Design review of the part built by this model. Coordinates are the model's own, in mm. Face numbers are marked on the shaded views. A direction names the side the tool comes from. Round coordinates to 2 decimals unless told otherwise and drop trailing zeros. Write each loop counter-clockwise with the first axis right and the second up, starting at its lowest first coordinate (ties: lowest second). Pieces come first, ordered by that corner, then holes. Notation, with made-up numbers: (62, 42.25) -> (117, 42.25) arc R14 ccw to (117, 59.25) -> close; hole circle Ø9 at (73, 60.5). An arc over 180 degrees is marked (long way). Write item = value, one per line. Start each with the question number.
Item 1: Mouldability with a two-part tool opening along X and no side actions: class the marked faces 3, 4, 5 and 6 as released by +X, released by -X, zero draft, split by the parting line, or undercut.
Item 2: Add section C-C, the plane z = 6.25. State how many separate pieces and enclosed holes the cut face has, then the cut area to 3 significant figures.
Item 3: To check wall thickness, follow L1, parallel to X at y = 20.4, z = 4.25; L2, parallel to X at y = 1.5, z = 6.75; L3, parallel to X at y = 19.5, z = 4.75. State the ranges of each line that lie inside material, in increasing order.
Item 4: Add section B-B, the plane y = -24.5. State the section outline as (x, z) points, then the cut area to 3 significant figures.
Item 5: Machinability: for the marked faces 1 and 2, which of the approach directions +Z, -Z, +X, -X, +Y, -Y give a long, thin tool a straight path to every point of the face, cutting with its end or side? Answer none if there is none.
Item 6: For pin 1 Ø2.5 at (x, y) = (27.2, -31.28) entering from +Z; pin 2 Ø4 at (x, z) = (-13.5, 4) entering from -Y; pin 3 Ø4.5 at (x, y) = (-28.5, 20.5) entering from +Z; pin 4 Ø1.5 at (x, y) = (0, -7) entering from -Z, all flat-tipped, find the tip position at first contact; note any pin that passes through.
Item 7: Add section A-A, the plane x = -4.5. State the section outline as (y, z) points, then the cut area to 3 significant figures.
from build123d import *

# Parameters (mm, degrees)
SKETCH2_R           = 1.5
BOSS_EXTRUDE1_DEPTH = 10.35
BOSS_EXTRUDE2_START = 10.35
SKETCH2_3_R         = 1.5
BOSS_EXTRUDE2_DEPTH = 3
FILLET1_SIZE        = 4
FILLET2_SIZE        = 4
SKETCH7_R           = 2.825
CUT_EXTRUDE1_DEPTH  = 3.5


with BuildPart() as part:
    # Sketch2 → Boss-Extrude1 (new body)
    with BuildSketch(Plane.XY):
        Polygon((-30.92, -35), (-23.9, -35), (-23.9, 18.9), (23.9, 18.9), (23.9, -35), (30.92, -35), (30.92, 24.12), (-30.92, 24.12), align=None)
        with Locations((-27.2, -31.28)):
            Circle(SKETCH2_R, mode=Mode.SUBTRACT)
        with Locations((27.2, -31.28)):
            Circle(SKETCH2_R, mode=Mode.SUBTRACT)
        with Locations((-27.2, 20.4)):
            Circle(SKETCH2_R, mode=Mode.SUBTRACT)
        with Locations((27.2, 20.4)):
            Circle(SKETCH2_R, mode=Mode.SUBTRACT)
    extrude(amount=BOSS_EXTRUDE1_DEPTH)

    # Sketch2<3> → Boss-Extrude2 (add)
    # profile 1 of 2: a face of its own
    with BuildSketch(Plane.XY.offset(BOSS_EXTRUDE2_START)):
        Polygon((-30.92, -35), (-23.9, -35), (-23.9, 18.9), (23.9, 18.9), (23.9, -35), (30.92, -35), (30.92, 24.12), (-30.92, 24.12), align=None)
        with Locations((-27.2, -31.28)):
            Circle(SKETCH2_3_R, mode=Mode.SUBTRACT)
        with Locations((27.2, -31.28)):
            Circle(SKETCH2_3_R, mode=Mode.SUBTRACT)
        with Locations((-27.2, 20.4)):
            Circle(SKETCH2_3_R, mode=Mode.SUBTRACT)
        with Locations((27.2, 20.4)):
            Circle(SKETCH2_3_R, mode=Mode.SUBTRACT)
    # profile 2 of 2: a face of its own
    with BuildSketch(Plane.XY.offset(BOSS_EXTRUDE2_START)):
        Polygon((-23.9, -35), (-16, -35), (16, -35), (23.9, -35), (23.9, 18.9), (-23.9, 18.9), align=None)
    extrude(amount=BOSS_EXTRUDE2_DEPTH)

    # Fillet1
    # a fillet whose section is not a circle: 4 mm, written as the material it adds along each edge
    with BuildSketch(Plane(origin=(-23.9, 18.9, 0), x_dir=(0, -1, 0), z_dir=(0, 0, 1))) as fillet1_piece_1_section:
        with BuildLine():
            add(Edge.make_bspline([(FILLET1_SIZE, 0), (FILLET1_SIZE * 0.831801948466, 0), (FILLET1_SIZE * 0.663603896932, 0), (FILLET1_SIZE * 0.292893218813, FILLET1_SIZE * 0.0716919198361), (FILLET1_SIZE * 0.0716919198361, FILLET1_SIZE * 0.292893218813), (0, FILLET1_SIZE * 0.663603896932), (0, FILLET1_SIZE * 0.831801948466), (0, FILLET1_SIZE)], knots=[0, 0, 0, 0, 0, 0, 0.5, 0.5, 1, 1, 1, 1, 1, 1], degree=5))
            Line((0, FILLET1_SIZE), (0, 0))
            Line((0, 0), (FILLET1_SIZE, 0))
        make_face()
    fillet1_piece_1 = extrude(amount=20.35, mode=Mode.PRIVATE)
    fillet1_piece_1 = split(fillet1_piece_1, bisect_by=Plane(origin=(-23.9, 18.9, 13.35), z_dir=(0, 0, -1)), keep=Keep.TOP, mode=Mode.PRIVATE)
    add(fillet1_piece_1)
    with BuildSketch(Plane(origin=(23.9, 18.9, 0), x_dir=(-1, 0, 0), z_dir=(0, 0, 1))) as fillet1_piece_2_section:
        with BuildLine():
            add(Edge.make_bspline([(FILLET1_SIZE, 0), (FILLET1_SIZE * 0.831801948466, 0), (FILLET1_SIZE * 0.663603896932, 0), (FILLET1_SIZE * 0.292893218813, FILLET1_SIZE * 0.0716919198361), (FILLET1_SIZE * 0.0716919198361, FILLET1_SIZE * 0.292893218813), (0, FILLET1_SIZE * 0.663603896932), (0, FILLET1_SIZE * 0.831801948466), (0, FILLET1_SIZE)], knots=[0, 0, 0, 0, 0, 0, 0.5, 0.5, 1, 1, 1, 1, 1, 1], degree=5))
            Line((0, FILLET1_SIZE), (0, 0))
            Line((0, 0), (FILLET1_SIZE, 0))
        make_face()
    fillet1_piece_2 = extrude(amount=20.35, mode=Mode.PRIVATE)
    fillet1_piece_2 = split(fillet1_piece_2, bisect_by=Plane(origin=(23.9, 18.9, 13.35), z_dir=(0, 0, -1)), keep=Keep.TOP, mode=Mode.PRIVATE)
    add(fillet1_piece_2)

    # Fillet2
    # a fillet whose section is not a circle: 4 mm, written as the material it takes off along each edge
    with BuildSketch(Plane(origin=(23.9, -35, -10), x_dir=(0, 1, 0), z_dir=(0, 0, 1)), Plane(origin=(-23.9, -35, -10), x_dir=(-1, 0, 0), z_dir=(0, 0, 1))) as fillet2_piece_1:
        with BuildLine():
            add(Edge.make_bspline([(FILLET2_SIZE, 0), (FILLET2_SIZE * 0.831801948466, 0), (FILLET2_SIZE * 0.663603896932, 0), (FILLET2_SIZE * 0.292893218813, -FILLET2_SIZE * 0.0716919198361), (FILLET2_SIZE * 0.0716919198361, -FILLET2_SIZE * 0.292893218813), (0, -FILLET2_SIZE * 0.663603896932), (0, -FILLET2_SIZE * 0.831801948466), (0, -FILLET2_SIZE)], knots=[0, 0, 0, 0, 0, 0, 0.5, 0.5, 1, 1, 1, 1, 1, 1], degree=5))
            Line((0, -FILLET2_SIZE), (0, 0))
            Line((0, 0), (FILLET2_SIZE, 0))
        make_face()
    extrude(amount=20.35, mode=Mode.SUBTRACT)
    with BuildSketch(Plane(origin=(-30.92, -35, 23.35), x_dir=(1, 0, 0), z_dir=(0, 0, -1)), Plane(origin=(30.92, -35, -10), x_dir=(-1, 0, 0), z_dir=(0, 0, 1))) as fillet2_piece_2:
        with BuildLine():
            add(Edge.make_bspline([(FILLET2_SIZE, 0), (FILLET2_SIZE * 0.831801948466, 0), (FILLET2_SIZE * 0.663603896932, 0), (FILLET2_SIZE * 0.292893218813, -FILLET2_SIZE * 0.0716919198361), (FILLET2_SIZE * 0.0716919198361, -FILLET2_SIZE * 0.292893218813), (0, -FILLET2_SIZE * 0.663603896932), (0, -FILLET2_SIZE * 0.831801948466), (0, -FILLET2_SIZE)], knots=[0, 0, 0, 0, 0, 0, 0.5, 0.5, 1, 1, 1, 1, 1, 1], degree=5))
            Line((0, -FILLET2_SIZE), (0, 0))
            Line((0, 0), (FILLET2_SIZE, 0))
        make_face()
    extrude(amount=33.35, mode=Mode.SUBTRACT)
    with BuildSketch(Plane(origin=(30.92, 24.12, 23.35), x_dir=(0, -1, 0), z_dir=(0, 0, -1)), Plane(origin=(-30.92, 24.12, 23.35), x_dir=(1, 0, 0), z_dir=(0, 0, -1))) as fillet2_piece_3:
        with BuildLine():
            add(Edge.make_bspline([(FILLET2_SIZE, 0), (FILLET2_SIZE * 0.831801948466, 0), (FILLET2_SIZE * 0.663603896932, 0), (FILLET2_SIZE * 0.292893218813, FILLET2_SIZE * 0.0716919198361), (FILLET2_SIZE * 0.0716919198361, FILLET2_SIZE * 0.292893218813), (0, FILLET2_SIZE * 0.663603896932), (0, FILLET2_SIZE * 0.831801948466), (0, FILLET2_SIZE)], knots=[0, 0, 0, 0, 0, 0, 0.5, 0.5, 1, 1, 1, 1, 1, 1], degree=5))
            Line((0, FILLET2_SIZE), (0, 0))
            Line((0, 0), (FILLET2_SIZE, 0))
        make_face()
    extrude(amount=33.35, mode=Mode.SUBTRACT)

    # Sketch7 → Cut-Extrude1 (cut)
    with BuildSketch(Plane.XY.offset(13.35)):
        with Locations((-27.2, 20.4)):
            Circle(SKETCH7_R)
        with Locations((27.2, 20.4)):
            Circle(SKETCH7_R)
        with Locations((27.2, -31.28)):
            Circle(SKETCH7_R)
        with Locations((-27.2, -31.28)):
            Circle(SKETCH7_R)
    extrude(amount=-CUT_EXTRUDE1_DEPTH, mode=Mode.SUBTRACT)


solid = part.part
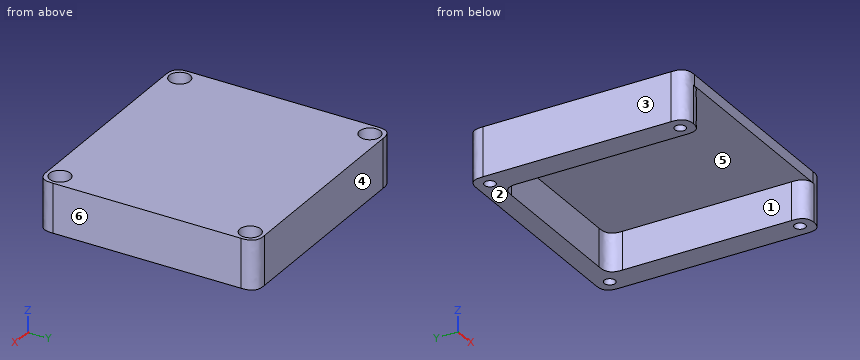
Result set:
q1.face_3 = released by -X
q1.face_4 = zero draft
q1.face_5 = undercut
q1.face_6 = released by +X
q2.separate_pieces = 1
q2.enclosed_holes = 4
q2.area = 1,040 mm²
q3.L1 = -30.92 to -28.7, -25.7 to 25.7, 28.7 to 30.92
q3.L2 = -30.92 to -23.9, 23.9 to 30.92
q3.L3 = -30.92 to -28.4, -26 to 26, 28.4 to 30.92
q4.outline = (-30.92, 0) -> (-23.9, 0) -> (-23.9, 10.35) -> (23.9, 10.35) -> (23.9, 0) -> (30.92, 0) -> (30.92, 13.35) -> (-30.92, 13.35) -> close
q4.area = 331 mm²
q5.face_1 = -Z, -Y
q5.face_2 = -Z, +X, -X, +Y, -Y
q6.pin_1 = through
q6.pin_2 = 18.9
q6.pin_3 = 13.35
q6.pin_4 = 10.35
q7.outline = (-35, 10.35) -> (18.9, 10.35) -> (18.9, 0) -> (24.12, 0) -> (24.12, 13.35) -> (-35, 13.35) -> close
q7.area = 231 mm²
